from build123d import *

# Parameters (mm, degrees)
CUT_EXTRUDE1_START  = 2.655
CUT_EXTRUDE1_DEPTH  = 10.16
CIRPATTERN1_COUNT   = 16
SKETCH4_R           = 1.7526
CUT_EXTRUDE2_DEPTH  = 16.477114557
CUT_EXTRUDE3_DEPTH  = 1.31445
CIRPATTERN3_COUNT   = 2
CIRPATTERN3_ANGLE   = 90
CHAMFER1_SIZE       = 0.28075
CUT_EXTRUDE4_START  = -6.12
SKETCH7_R           = 9.015
CUT_EXTRUDE4_DEPTH  = 6.12
SKETCH8_R           = 2.475
CUT_EXTRUDE5_DEPTH  = 18.122656044
SKETCH9_R           = 3.75
SKETCH9_R_2         = 2.475
BOSS_EXTRUDE1_DEPTH = 1.35


with BuildPart() as part:
    # Sketch2 → Revolve1 (revolve)
    with BuildSketch(Plane(origin=(0, 0, 0), x_dir=(0, 0, -1), z_dir=(1, 0, 0)), mode=Mode.PRIVATE) as revolve1_sk:
        Polygon((-8.775, 2.38125), (8.775, 2.38125), (8.775, 9.015), (8.14, 9.015), (7.505, 8.13975), (7.505, 7.2645), (-2.655, 7.2645), (-2.655, 8.13975), (-3.29, 9.015), (-8.775, 9.015), align=None)
    revolve(revolve1_sk.sketch.rotate(Axis((0, 0, 8.775), (0, 0, -1)), 90), axis=Axis((0, 0, 8.775), (0, 0, -1)))

    # Sketch3 → Cut-Extrude1 (cut)
    with BuildSketch(Plane.XY.offset(CUT_EXTRUDE1_START)):
        with BuildLine():
            Line((3.757926927, 9.015), (-3.757926927, 9.015))
            Line((-3.757926927, 9.015), (-2.795101196, 6.705249403))
            ThreePointArc((-2.795101196, 6.705249403), (-1.995846132, 6.984952288), (-1.169472895, 7.169748489))
            ThreePointArc((-1.169472895, 7.169748489), (-0.985767742, 7.127751824), (-0.883573242, 6.969424355))
            ThreePointArc((-0.883573242, 6.969424355), (-0.839120956, 6.792881518), (-0.773880597, 6.622919538))
            ThreePointArc((-0.773880597, 6.622919538), (0, 6.1245), (0.773880597, 6.622919538))
            ThreePointArc((0.773880597, 6.622919538), (0.839120956, 6.792881518), (0.883573242, 6.969424355))
            ThreePointArc((0.883573242, 6.969424355), (0.985767742, 7.127751824), (1.169472895, 7.169748489))
            ThreePointArc((1.169472895, 7.169748489), (1.995846132, 6.984952288), (2.795101196, 6.705249403))
            Line((2.795101196, 6.705249403), (3.757926927, 9.015))
        make_face()
    cut_extrude1 = extrude(amount=-CUT_EXTRUDE1_DEPTH, mode=Mode.SUBTRACT)

    # CirPattern1: Cut-Extrude1 ×16 about axis
    cirpattern1_axis = Axis((0, 0, 0), (0, 0, 1))
    for i in range(1, CIRPATTERN1_COUNT):
        add(cut_extrude1.rotate(cirpattern1_axis, i * 360 / CIRPATTERN1_COUNT), mode=Mode.SUBTRACT)

    # Sketch4 → Cut-Extrude2 (cut, through all)
    with BuildSketch(Plane(origin=(0, 0, 0), x_dir=(0, -1, 0), z_dir=(1, 0, 0))):
        with Locations(Location((0, -5.715, 0), (0, 0, 270))):
            Circle(SKETCH4_R)
    cut_extrude2 = extrude(amount=CUT_EXTRUDE2_DEPTH, mode=Mode.SUBTRACT)

    # Sketch5 → Revolve2 (revolve)
    with BuildSketch(Plane.XY.offset(5.715), mode=Mode.PRIVATE) as revolve2_sk:
        Polygon((2.38125, -1.3716), (2.38125, 0), (8.842998261, 0), (8.842998261, -1.3716), (8.461998261, -1.7526), (2.76225, -1.7526), align=None)
    revolve2 = revolve(revolve2_sk.sketch.rotate(Axis((2.38125, 0, 5.715), (1, 0, 0)), 270), axis=Axis((2.38125, 0, 5.715), (1, 0, 0)))

    # Sketch6 → Cut-Extrude3 (cut)
    with BuildSketch(Plane(origin=(8.842998261, 5.384140679, 0), x_dir=(0, -1, 0), z_dir=(-1, 0, 0))):
        Polygon((5.384140679, 6.726864082), (4.507840679, 6.220932041), (4.507840679, 5.209067959), (5.384140679, 4.703135918), (6.260440679, 5.209067959), (6.260440679, 6.220932041), align=None)
    cut_extrude3 = extrude(amount=CUT_EXTRUDE3_DEPTH, mode=Mode.SUBTRACT)

    # CirPattern3: Cut-Extrude2, Revolve2, Cut-Extrude3 ×2 about axis
    cirpattern3_axis = Axis((0, 0, 0), (0, 0, 1))
    add([cut_extrude2.rotate(cirpattern3_axis, i * CIRPATTERN3_ANGLE / (CIRPATTERN3_COUNT - 1)) for i in range(1, CIRPATTERN3_COUNT)], mode=Mode.SUBTRACT)
    add([revolve2.rotate(cirpattern3_axis, i * CIRPATTERN3_ANGLE / (CIRPATTERN3_COUNT - 1)) for i in range(1, CIRPATTERN3_COUNT)])
    add([cut_extrude3.rotate(cirpattern3_axis, i * CIRPATTERN3_ANGLE / (CIRPATTERN3_COUNT - 1)) for i in range(1, CIRPATTERN3_COUNT)], mode=Mode.SUBTRACT)

    # Chamfer1
    chamfer1_edges = [part.edges().sort_by_distance(p)[0] for p in [
        (-2.38125, 0, 8.775),
        (-9.015, 0, 8.775),
    ]]
    chamfer(chamfer1_edges, length=CHAMFER1_SIZE)

    # Sketch7 → Cut-Extrude4 (cut)
    with BuildSketch(Plane.XY.offset(8.775).offset(CUT_EXTRUDE4_START)):
        Circle(SKETCH7_R)
    extrude(amount=CUT_EXTRUDE4_DEPTH, mode=Mode.SUBTRACT)

    # Sketch8 → Cut-Extrude5 (cut, through all)
    with BuildSketch(Plane(origin=(0, 0, -8.775), x_dir=(-1, 0, 0), z_dir=(0, 0, -1))):
        Circle(SKETCH8_R)
    extrude(amount=-CUT_EXTRUDE5_DEPTH, mode=Mode.SUBTRACT)

    # Sketch9 → Boss-Extrude1 (add)
    with BuildSketch(Plane.XY.offset(2.655)):
        with Locations(Location((0, 0, 0), (0, 0, 180))):
            Circle(SKETCH9_R)
        with Locations(Location((0, 0, 0), (0, 0, 180))):
            Circle(SKETCH9_R_2, mode=Mode.SUBTRACT)
    extrude(amount=BOSS_EXTRUDE1_DEPTH)


solid = part.part
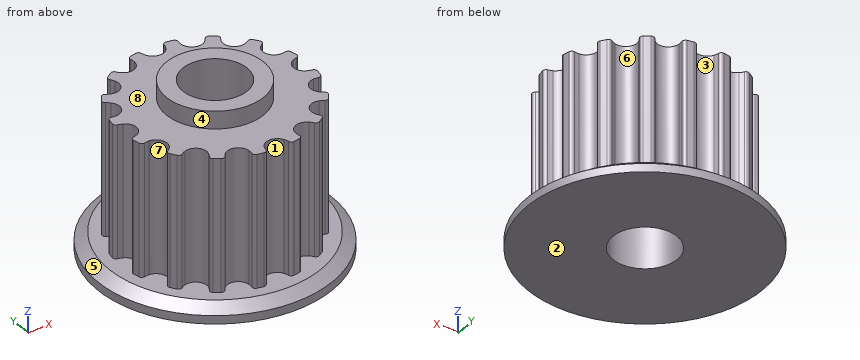
Source: CAD feature listing. Evaluate the final solid. Frame: model axes, mm. Face numbers are marked on the shaded views. A direction names the side the tool comes from. Coordinates: 2 decimals unless noted, no trailing zeros.
Item 1: Material intervals for line 1 (X direction, y = 0, z = 0) (1 decimal); line 2 (Z direction, x = -6, y = -2.5) (3 decimals), sorted ascending.
Output values:
line 1: x = -6.1 to -2.5, 2.5 to 6.1
line 2: z = -8.775 to -7.505
Item 2: First-contact query: P1, Ø1.5, axis at y = 3.5, z = -5, coming from the -X side; P2, Ø1, axis at x = 0.5, y = -4.5, coming from the +Z side (3 decimals); P3, Ø5, axis at x = 3.5, z = 0, coming from the -Y side; P4, Ø4, axis at x = 0, y = 0, coming from the -Z side. Flat tips, straight axial feed; report the tip coordinate or a pass-through.
Output values:
P1: stops at x = -6.21
P2: stops at z = 2.655
P3: stops at y = -7.17
P4: passes through
Item 3: Pull-direction query (Y, two-part tool) for the marked faces 5, 6, 7 and 8; classes: pulls with the +Y half, pulls with the -Y half, needs draft (parallel to the pull), parting line crosses it, or undercut.
Output values:
face 5: parting line crosses it
face 6: undercut
face 7: undercut
face 8: needs draft
Item 4: Set-up query: the marked faces 1, 2, 3 and 4. Return all of +Z, -Z, +X, -X, +Y, -Y with unobstructed straight access to the full face (end or side cutting, diameter ignored); none if empty.
Output values:
face 1: +Z, -Y
face 2: -Z, +X, -X, +Y, -Y
face 3: +Z, +Y
face 4: +Z
